from build123d import *

# Parameters (mm, degrees)
F0_R     = 50
F0_R_2   = 45
F1_DEPTH = 100
F2_R     = 45
F3_DEPTH = 12.954
F4_R     = 7.5
F5_DEPTH = 12.954
F6_R     = 10
F6_R_2   = 7.5
F7_DEPTH = 100


with BuildPart() as f1:
    # F0 (on Top) → F1 (new body)
    with BuildSketch(Plane.XY):
        Circle(F0_R)
        Circle(F0_R_2, mode=Mode.SUBTRACT)
    extrude(amount=F1_DEPTH)

    # F2 (on face) → F3 (join)
    with BuildSketch(Plane(origin=(0, 0, 0), x_dir=(1, 0, 0), z_dir=(0, 0, -1))):
        Circle(F2_R)
    extrude(amount=-F3_DEPTH)

    # F4 (on face) → F5 (cut, through all)
    with BuildSketch(Plane(origin=(0, 0, 0), x_dir=(1, 0, 0), z_dir=(0, 0, -1))):
        Circle(F4_R)
    extrude(amount=-F5_DEPTH, mode=Mode.SUBTRACT)

    # F6 (on face) → F7 (join)
    with BuildSketch(Plane(origin=(0, 0, 0), x_dir=(1, 0, 0), z_dir=(0, 0, -1))):
        Circle(F6_R)
        Circle(F6_R_2, mode=Mode.SUBTRACT)
    extrude(amount=F7_DEPTH)


solid = f1.part
Here's how the part is built. I have some questions about the finished solid (model axes, mm). A direction names the side the tool comes from. Coordinates: 2 decimals unless noted, no trailing zeros. Write each loop counter-clockwise with the first axis right and the second up, starting at its lowest first coordinate (ties: lowest second). Pieces come first, ordered by that corner, then holes.
Item 1: I want a section at A-A on y = 0. Write out the boundary of the cut face in (x, z), and give its area (3 significant figures).
Item 2: On a 3-axis mill with a long thin cutter (end or side, diameter ignored), from which of +Z, -Z, +X, -X, +Y, -Y can I reach the whole of each face in a straight line? I mean faces 1 (the cylindrical face through (20.765, -39.923, 55.868)), 2 (the cylindrical face through (-2.17, 9.76, -49.3)), 3 (the flat face through (-41, 19, 100)). Say none if no direction works.
Item 3: If we mould it in two halves opening along X, with no side actions, what happens to faces 4 (the cylindrical face through (47.69, 15.02, 49.3)), 5 (the flat face through (4, -7, -100)), 6 (the cylindrical face through (-7.493, -0.33, -42.732)), 7 (the flat face through (-1, 9, 12.954))? For each: +X half, -X half, draft (parallel to the pull), parting line (faces both ways), or undercut.
Item 4: Will these pins go through, and if not, where does the flat tip stop? pin 1 (4 mm diameter, centred on x = 37.5, y = 16.5, fed in from -Z); pin 2 (1 mm diameter, centred on x = 19, z = 73.5, fed in from +Y); pin 3 (12 mm diameter, centred on x = 0, y = 0, fed in from -Z); pin 4 (2 mm diameter, centred on x = 9.5, y = -31.5, fed in from +Z).
Item 5: If I drill on line 1 (Y direction, x = 0, z = 77); line 2 (Z direction, x = 37.5, y = -1); line 3 (X direction, y = 15, z = 60.5), over which ranges is the centre line in solid material (lowest first)?
Item 6: I want a section at C-C on z = -3.5. Write out the boundary of the cut face in (x, y).
Item 7: I want a section at D-D on y = -16. Write out the boundary of the cut face in (x, z).
Findings below:
1. outline: (-50, 0) - (-10, 0) - (-10, -100) - (-7.5, -100) - (-7.5, 12.95) - (-45, 12.95) - (-45, 100) - (-50, 100) - close; (7.5, -100) - (10, -100) - (10, 0) - (50, 0) - (50, 100) - (45, 100) - (45, 12.95) - (7.5, 12.95) - close
1. area: 2,470 mm2
2. face 1: +Z
2. face 2: -Z
2. face 3: +Z, +X, -X, +Y, -Y
3. face 4: parting line
3. face 5: draft
3. face 6: undercut
3. face 7: undercut
4. pin 1: stops at z = 0
4. pin 2: stops at y = 46.45
4. pin 3: passes through
4. pin 4: stops at z = 12.95
5. line 1: y = -50 to -45, 45 to 50
5. line 2: z = 0 to 12.95
5. line 3: x = -47.7 to -42.43, 42.43 to 47.7
6. outline: circle Ø20 at (0, 0); hole circle Ø15 at (0, 0)
7. outline: (-47.37, 0) - (47.37, 0) - (47.37, 100) - (42.06, 100) - (42.06, 12.95) - (-42.06, 12.95) - (-42.06, 100) - (-47.37, 100) - close
